The listing builds one solid part. Answer for the finished solid, in the listing's coordinates (mm). A direction names the side the tool comes from. Give positions to 0.01 mm unless a question says otherwise; leave off trailing zeros. Write each loop counter-clockwise with the first axis right and the second up, starting at its lowest first coordinate (ties: lowest second). Pieces come first, ordered by that corner, then holes. Notation, with made-up numbers: M -23.5,-29 L -15.5,-29 A32 cw -15.5,4 Z; hole C -25,39.25 d7. An arc over 180 degrees is marked long. Return JSON: item names as keys, results as strings.
Autodesk Inventor part; units mm, degrees
ref_plane "Work Plane1" through (6.985, 0, 0) normal (1, 0, 0) x (0, 0, -1)
ref_plane "YZ Plane" through (0, 0, 0) normal (1, 0, 0) x (0, 1, 0)
ref_plane "XZ Plane" through (0, 0, 0) normal (0, 1, 0) x (-1, 0, 0)
sketch "Sketch1" plane through (0, 0, 0) normal (0, 0, 1) x (1, 0, 0)
  line L0 (0, -23.495) -> (13.97, -23.495)
  line L1 (0, 23.495) -> (0, -23.495)
  line L2 (13.97, -23.495) -> (13.97, 23.495)
  line L3 (2.54, -27.305) -> (-12.065, -27.305)
  line L4 (26.035, -27.305) -> (11.43, -27.305)
  line L5 (2.54, -31.115) -> (2.54, -27.305)
  line L6 (11.43, -27.305) -> (11.43, -31.115)
  line L7 (0, -31.115) -> (2.54, -31.115)
  line L8 (11.43, -31.115) -> (13.97, -31.115)
  line L9 (3.175, -36.449) -> (10.795, -36.449)
  line L10 (10.795, -36.449) -> (10.795, -28.7565)
  line L11 (3.175, -36.449) -> (3.175, -28.7565)
  line L12 (-2.794, -26.035) -> (0.4535, -26.035)
  line L13 (-0.254, -23.749) -> (14.224, -23.749)
  line L14 (14.224, -23.749) -> (14.224, -20.955)
  line L15 (14.224, -20.955) -> (16.764, -20.955)
  line L16 (16.764, -20.955) -> (16.764, -26.035)
  line L17 (16.764, -26.035) -> (13.5165, -26.035)
  arc A0 (3.175, -28.7565) -> (0.4535, -26.035) centre (0.4535, -28.7565) ccw
  arc A1 (13.5165, -26.035) -> (10.795, -28.7565) centre (13.5165, -28.7565) ccw
  line L18 (-19.685, 0) -> (33.655, 0)
  line L19 (-2.794, -26.035) -> (-2.794, -20.955)
  line L20 (-2.794, -20.955) -> (-0.254, -20.955)
  line L21 (-0.254, -20.955) -> (-0.254, -23.749)
  point P0 (0, 0)
  dimension "d0" = 0.635
  dimension "d1" = 0.635
  dimension "d2" = 7.62
  dimension "d3" = 0.254
  dimension "d4" = 0.254
  dimension "d5" = 2.54
  dimension "d6" = 2.54
  dimension "d7" = 1.27
  dimension "d9" = 12.7
  dimension "d10" = 2.5418
revolve "Revolution1" add sketch "Sketch1" angle 360 about axis through (-10, 0, 0) along (1, 0, 0) contours L11 A0 L12 L19 L20 L21 L13 L14 L15 L16 L17 A1 L10 L9
chamfer "Chamfer1" distance 1.27 angle 45 2 edges at (10.795, 36.449, 0) (3.175, 36.449, 0)
ref_plane "Work Plane1" through (6.985, 0, 0) normal (1, 0, 0) x (0, 0, -1)
sketch "Sketch2" plane through (6.985, 0, 0) normal (1, 0, 0) x (0, 0, -1)
  line L0 (58.906, -57.765) -> (-58.906, -57.765)
  line L1 (-58.906, -57.765) -> (-58.906, 57.765)
  line L2 (-58.906, 57.765) -> (58.906, 57.765)
  line L3 (58.906, 57.765) -> (58.906, -57.765)
  line L4 (58.906, -57.765) -> (-58.906, 57.765) construction
  line L5 (-58.906, -57.765) -> (58.906, 57.765) construction
  point P0 (0, 0)
extrude "Extrusion1" cut sketch "Sketch2" against normal through all
chamfer "Chamfer2" distance 1.27 angle 45 1 edges at (14.224, 23.749, 0)
equation "\"d1\" = d0"
equation "\"d4\" = d3"
properties part number "Big Bearing Cover"
Item 1: Find the intervals of material crossed by line 1 (Y direction, x = 15.55, z = 0) (3 decimals); line 2 (X direction, y = 15.5, z = 31.5) (3 decimals), in increasing order.
Geometry results:
{"line 1": "y = -26.035 to -20.955, 20.955 to 26.035", "line 2": "x = 6.985 to 10.795"}
Item 2: Determine the mould class of faces 4 (the flat face through (16.764, -1.8, -21.3)), 5 (the cylindrical face through (15.118, 3.389, 25.813)), 6 (the cylindrical face through (15.512, 2.728, -20.777)) for opening direction Z: +Z half, -Z half, draft (parallel to the pull), parting line (faces both ways), or undercut.
Geometry results:
{"face 4": "draft", "face 5": "parting line", "face 6": "undercut"}
Item 3: A cutting plane is placed at A-A, the plane y = 0. Write down the section's boundary in (x, z) (1 decimal), plus the area to 3 significant figures.
Geometry results:
{"outline": "M 7,-36.4 L 9.5,-36.4 L 10.8,-35.2 L 10.8,-28.8 A2.7 cw 13.5,-26 L 16.8,-26 L 16.8,-21 L 14.2,-21 L 14.2,-22.5 L 13,-23.7 L 7,-23.7 Z; M 7,23.7 L 13,23.7 L 14.2,22.5 L 14.2,21 L 16.8,21 L 16.8,26 L 13.5,26 A2.7 cw 10.8,28.8 L 10.8,35.2 L 9.5,36.4 L 7,36.4 Z", "area": "141 mm2"}
Item 4: Given pin 1 Ø1.5 at (x, y) = (10, -28.5) entering from +Z; pin 2 Ø4 at (x, z) = (10.5, -13) entering from -Y; pin 3 Ø3 at (x, z) = (15, -23) entering from +Y, each flat-ended and moving along its own axis, determine where each tip first touches the part or whether it passes through.
Geometry results:
{"pin 1": "stops at z = 23.43", "pin 2": "stops at y = -34.67", "pin 3": "stops at y = 14.68"}
Item 5: Which of the six approach directions +Z, -Z, +X, -X, +Y, -Y give full straight-line access (tool end or side, diameter ignored) to faces 1 (the cylindrical face through (8.273, 7.901, 35.582)), 2 (the flat face through (14.224, 7, 20)), 3 (the flat face through (10.795, 29, 0))?
Geometry results:
{"face 1": "+X, -X", "face 2": "-X", "face 3": "+X"}
